```python
from build123d import *

# Parameters (mm, degrees)
SKETCH1_R                = 15.5
BOSS_EXTRUDE1_DEPTH      = 60
SKETCH2_R                = 6
BOSS_EXTRUDE2_DEPTH      = 2
SKETCH3_W                = 27
SKETCH3_H                = 58
BOSS_EXTRUDE3_DEPTH      = 20
SKETCH4_R                = 9.5
BOSS_EXTRUDE4_DEPTH      = 3.5
BOSS_EXTRUDE5_START      = 3.5
SKETCH6_R                = 9.5
BOSS_EXTRUDE5_DEPTH      = 3.5
SKETCH7_R                = 4
BOSS_EXTRUDE6_DEPTH      = 15
CUT_EXTRUDE1_START       = -14
CUT_EXTRUDE1_DEPTH       = 14
BOSS_EXTRUDE7_DEPTH      = 2
BOSS_EXTRUDE7_DEPTH_BACK = 29
SKETCH10_R               = 3.8
F_4_0MM_DOWEL_HOLE1_D    = 4
FILLET1_R                = 3


with BuildPart() as part:
    # Sketch1 → Boss-Extrude1 (new body)
    with BuildSketch(Plane.XY):
        Circle(SKETCH1_R)
    extrude(amount=BOSS_EXTRUDE1_DEPTH)

    # Sketch2 → Boss-Extrude2 (add)
    with BuildSketch(Plane(origin=(0, 0, 0), x_dir=(-1, 0, 0), z_dir=(0, 0, -1))):
        Circle(SKETCH2_R)
    extrude(amount=BOSS_EXTRUDE2_DEPTH)

    # Sketch3 → Boss-Extrude3 (add, symmetric)
    with BuildSketch(Plane(origin=(0, 0, 0), x_dir=(1, 0, 0), z_dir=(0, 1, 0))):
        with Locations((-4.5, -89)):
            Rectangle(SKETCH3_W, SKETCH3_H)
    extrude(amount=BOSS_EXTRUDE3_DEPTH, both=True)

    # Sketch4 → Boss-Extrude4 (add)
    with BuildSketch(Plane.ZY.offset(18)):
        with Locations(Location((98, 0, 0), (0, 0, 180))):
            Circle(SKETCH4_R)
    extrude(amount=BOSS_EXTRUDE4_DEPTH)

    # Sketch6 → Boss-Extrude5 (add)
    with BuildSketch(Plane(origin=(9, 0, 0), x_dir=(0, 0, -1), z_dir=(1, 0, 0)).offset(BOSS_EXTRUDE5_START)):
        with Locations((-98, 0)):
            Circle(SKETCH6_R)
    extrude(amount=-BOSS_EXTRUDE5_DEPTH)

    # Sketch7 → Boss-Extrude6 (add)
    with BuildSketch(Plane.ZY.offset(21.5)):
        with Locations((98, 0)):
            Circle(SKETCH7_R)
    extrude(amount=BOSS_EXTRUDE6_DEPTH)

    # Sketch8 → Cut-Extrude1 (cut)
    with BuildSketch(Plane.ZY.offset(36.5).offset(CUT_EXTRUDE1_START)):
        with BuildLine():
            Line((101, 2.645751311), (101, -2.645751311))
            ThreePointArc((101, -2.645751311), (102, 0), (101, 2.645751311))
        make_face()
    extrude(amount=CUT_EXTRUDE1_DEPTH, mode=Mode.SUBTRACT)

    # Sketch10 → Boss-Extrude7 (add, two sides: drawn at the far end of the back side and taken through both)
    with BuildSketch(Plane(origin=(9, 0, 0), x_dir=(0, 0, -1), z_dir=(1, 0, 0)).offset(-BOSS_EXTRUDE7_DEPTH_BACK)):
        with Locations((-69, 14)):
            Circle(SKETCH10_R)
        with Locations((-109, 14)):
            Circle(SKETCH10_R)
        with Locations((-69, -14)):
            Circle(SKETCH10_R)
        with Locations((-109, -14)):
            Circle(SKETCH10_R)
    extrude(amount=BOSS_EXTRUDE7_DEPTH + BOSS_EXTRUDE7_DEPTH_BACK)

    # Ø4.0mm Dowel Hole1 (through all)
    with Locations(Plane(origin=(11, 0, 0), x_dir=(0, 0, -1), z_dir=(1, 0, 0))):
        with Locations((-109, 14), (-69, 14), (-69, -14), (-109, -14)):
            Hole(F_4_0MM_DOWEL_HOLE1_D / 2)

    # Fillet1
    fillet1_edges = [part.edges().sort_by_distance(p)[0] for p in [
        (-4.5, -20, 60),
        (-4.5, -20, 118),
        (-4.5, 20, 60),
        (-4.5, 20, 118),
    ]]
    fillet(fillet1_edges, radius=FILLET1_R)


solid = part.part
```
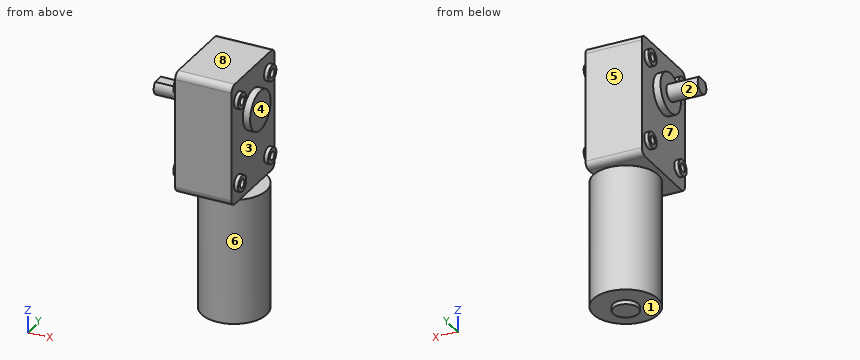
Could you check a few things on this model? Use its own coordinates, in mm. Face numbers are marked on the shaded views. A direction names the side the tool comes from. Give positions to 0.01 mm unless a question says otherwise; leave off trailing zeros. Loops run counter-clockwise (first coordinate to the right, second up) from the corner with the lowest first, then second, coordinate; pieces in that order, holes last. Notation, with made-up numbers: (-23.75, -27.5) - (6.25, -27.5) arc R16 ccw to (6.25, -15.5) - close; hole circle Ø5 at (-28.5, -27). An arc over 180 degrees is marked (long way). Answer in a Markdown table with one row per item. Add a question column.
Q1. Which directions (+Z, -Z, +X, -X, +Y, -Y) give clear straight access to the entire face, cutting with the end or side of a thin tool? Please do the marked faces 1, 2, 3, 4 and 5.
Q2. We'd pull the mould along Z, two halves only. Please class the marked faces 6, 7 and 8: +Z half, -Z half, draft (parallel to the pull), parting line (faces both ways), or undercut.
Q3. If we section it at A-A (z = 109): List the corners of the cut face in (x, y) for me, plus the area to 3 significant figures.
Q4. If we section it at B-B (x = 0): List the corners of the cut face in (y, z) for me.
Q5. For pin 1 (4 mm diameter, centred on y = 14.5, z = 70.5, fed in from -X); pin 2 (8.5 mm diameter, centred on y = 12.5, z = 69.5, fed in from +X); pin 3 (1 mm diameter, centred on x = -7.5, y = 13, fed in from -Z), each with a flat end and sliding along its axis, tell me the tip position at first contact or that it passes through.
Q6. Please list where these lines run through material, in increasing order: L1, parallel to Y at x = -9.5, z = 109; L2, parallel to Z at x = -2, y = -15.5; L3, parallel to X at y = 13.5, z = 85. Write a range as from..to.
Q7. If we section it at D-D (x = -27): List the corners of the cut face in (y, z) for me.
Q8. If we section it at C-C (y = -14): State how many separate pieces and enclosed holes the cut face has, plus the area to 3 significant figures.
The answers:
| question | item | result |
|---|---|---|
| 1 | face 1 | -Z |
| 1 | face 2 | -X |
| 1 | face 3 | +X |
| 1 | face 4 | +Z, +X, +Y, -Y |
| 1 | face 5 | +Z, -Z, +X, -X, +Y |
| 2 | face 6 | draft |
| 2 | face 7 | undercut |
| 2 | face 8 | +Z half |
| 3 | outline | (-20, -17.8) - (-18, -17.8) - (-18, -20) - (9, -20) - (9, -17.8) - (11, -17.8) - (11, -16) - (-20, -16) - close; (-20, -12) - (11, -12) - (11, -10.2) - (9, -10.2) - (9, 10.2) - (11, 10.2) - (11, 12) - (-20, 12) - (-20, 10.2) - (-18, 10.2) - (-18, -10.2) - (-20, -10.2) - close; (-20, 16) - (11, 16) - (11, 17.8) - (9, 17.8) - (9, 20) - (-18, 20) - (-18, 17.8) - (-20, 17.8) - close |
| 3 | area | 893 mm^2 |
| 4 | outline | (-20, 63) arc R3 ccw to (-17, 60) - (-15.5, 60) - (-15.5, 0) - (-6, 0) - (-6, -2) - (6, -2) - (6, 0) - (15.5, 0) - (15.5, 60) - (17, 60) arc R3 ccw to (20, 63) - (20, 115) arc R3 ccw to (17, 118) - (-17, 118) arc R3 ccw to (-20, 115) - close; hole circle Ø4 at (-14, 69); hole circle Ø4 at (-14, 109); hole circle Ø4 at (14, 69); hole circle Ø4 at (14, 109) |
| 5 | pin 1 | stops at x = -20 |
| 5 | pin 2 | stops at x = 11 |
| 5 | pin 3 | stops at z = 0 |
| 6 | L1 | y = -20..-16, -12..12, 16..20 |
| 6 | L2 | z = 60..67.68, 70.32..107.68, 110.32..118 |
| 6 | L3 | x = -18..9 |
| 7 | outline | (-2.65, 101) arc R4 ccw (long way) to (2.65, 101) - close |
| 8 | separate pieces | 3 |
| 8 | enclosed holes | 0 |
| 8 | area | 2,180 mm^2 |
